from build123d import *

# Parameters (mm, degrees)
WYCI_GNI_CIE1_DEPTH        = 62
SZKIC2_R                   = 2.125
WYTNIJ_WYCI_GNI_CIE1_DEPTH = 21
SZKIC3_R                   = 2.7
WYTNIJ_WYCI_GNI_CIE2_DEPTH = 16
SZKIC4_W                   = 5
SZKIC4_H                   = 2
WYTNIJ_WYCI_GNI_CIE3_DEPTH = 21
SFAZOWANIE1_SIZE           = 0.5
SZKIC5_R                   = 2.5
WYTNIJ_WYCI_GNI_CIE4_DEPTH = 16
SZKIC6_R                   = 4
WYTNIJ_WYCI_GNI_CIE5_DEPTH = 5
SZKIC7_R                   = 2.5
WYTNIJ_WYCI_GNI_CIE6_DEPTH = 10


with BuildPart() as part:
    # Szkic1 → Wyciągnięcie1 (new body)
    with BuildSketch(Plane(origin=(0, 0, 0), x_dir=(0, 0, -1), z_dir=(1, 0, 0))):
        Polygon((0, 0), (0, -20), (13, -20), (13, -15), (15, -15), (15, -5), (13, -5), (13, 0), align=None)
    extrude(amount=WYCI_GNI_CIE1_DEPTH)

    # Szkic2 → Wytnij-wyciągnięcie1 (cut, through all)
    with BuildSketch(Plane(origin=(0, 0, 0), x_dir=(-1, 0, 0), z_dir=(0, 1, 0))):
        with Locations((-7.75, 0)):
            Circle(SZKIC2_R)
        with Locations((-23.25, 0)):
            Circle(SZKIC2_R)
        with Locations((-38.75, 0)):
            Circle(SZKIC2_R)
        with Locations((-54.25, 0)):
            Circle(SZKIC2_R)
    extrude(amount=-WYTNIJ_WYCI_GNI_CIE1_DEPTH, mode=Mode.SUBTRACT)

    # Szkic3 → Wytnij-wyciągnięcie2 (cut)
    with BuildSketch(Plane(origin=(0, -2, 0), x_dir=(-1, 0, 0), z_dir=(0, 1, 0))):
        with Locations((-7.75, 0)):
            Circle(SZKIC3_R)
        with Locations((-23.25, 0)):
            Circle(SZKIC3_R)
        with Locations((-38.75, 0)):
            Circle(SZKIC3_R)
        with Locations((-54.25, 0)):
            Circle(SZKIC3_R)
    extrude(amount=-WYTNIJ_WYCI_GNI_CIE2_DEPTH, mode=Mode.SUBTRACT)

    # Szkic4 → Wytnij-wyciągnięcie3 (cut, through all)
    with BuildSketch(Plane(origin=(0, 0, 0), x_dir=(-1, 0, 0), z_dir=(0, 1, 0))):
        with Locations((-59.5, -14)):
            Rectangle(SZKIC4_W, SZKIC4_H)
        with Locations((-2.5, -14)):
            Rectangle(SZKIC4_W, SZKIC4_H)
    extrude(amount=-WYTNIJ_WYCI_GNI_CIE3_DEPTH, mode=Mode.SUBTRACT)

    # Sfazowanie1
    sfazowanie1_edges = [part.edges().sort_by_distance(p)[0] for p in [
        (31, -5, -15),
        (31, -15, -15),
        (57, -10, -15),
        (31, 0, -13),
        (62, -10, -13),
        (31, -20, -13),
        (5, -10, -15),
        (0, -10, -13),
    ]]
    chamfer(sfazowanie1_edges, length=SFAZOWANIE1_SIZE)

    # Szkic5 → Wytnij-wyciągnięcie4 (cut, through all)
    with BuildSketch(Plane.XY):
        with Locations((31, -10)):
            Circle(SZKIC5_R)
        with Locations((46.5, -10)):
            Circle(SZKIC5_R)
        with Locations((15.5, -10)):
            Circle(SZKIC5_R)
    extrude(amount=-WYTNIJ_WYCI_GNI_CIE4_DEPTH, mode=Mode.SUBTRACT)

    # Szkic6 → Wytnij-wyciągnięcie5 (cut)
    with BuildSketch(Plane.XY):
        with Locations((46.5, -10)):
            Circle(SZKIC6_R)
        with Locations((31, -10)):
            Circle(SZKIC6_R)
        with Locations((15.5, -10)):
            Circle(SZKIC6_R)
    extrude(amount=-WYTNIJ_WYCI_GNI_CIE5_DEPTH, mode=Mode.SUBTRACT)

    # Szkic7 → Wytnij-wyciągnięcie6 (cut)
    with BuildSketch(Plane.XZ.offset(20)):
        with Locations((7.75, 0)):
            Circle(SZKIC7_R)
        with Locations((23.25, 0)):
            Circle(SZKIC7_R)
        with Locations((38.75, 0)):
            Circle(SZKIC7_R)
        with Locations((54.25, 0)):
            Circle(SZKIC7_R)
    extrude(amount=-WYTNIJ_WYCI_GNI_CIE6_DEPTH, mode=Mode.SUBTRACT)


solid = part.part
For this review, take the finished solid that the model builds, in its own axes (mm). A direction names the side the tool comes from. Give positions to 0.01 mm unless a question says otherwise; leave off trailing zeros. Order: outer loops, then holes, each group sorted by start corner. A loop starts at its lowest first (then second) coordinate and runs counter-clockwise, first axis right, second up. Notation, with made-up numbers: (85.25, 87.5) - (137.25, 87.5) arc R24 cw to (137.25, 126.5) - close; hole circle Ø7 at (40.5, -22.75). An arc over 180 degrees is marked (long way). Answer as a JSON object with one key per item and string values. Group by question number.
Item 1: Take a section at B-B on x = 15.5. Give the boundary of the cut face in (y, z), and give its area (4 significant figures).
Item 2: Take a section at A-A on z = -9.25. Give the boundary of the cut face in (x, y).
Item 3: Clearance check with flat-ended pins moving along their axes: pin 1 Ø0.8 at (y, z) = (-10, -13.5) entering from +X; pin 2 Ø1.6 at (x, z) = (35, -13.5) entering from +Y; pin 3 Ø2 at (x, z) = (23, -1) entering from -Y. State where each tip first meets the part, or that it passes through.
Item 4: Take a section at D-D on x = 54.25. Give the boundary of the cut face in (y, z) (3 decimals), and give its area (3 significant figures).
Item 5: Take a section at C-C on y = -16. Give the boundary of the cut face in (x, z), and give its area (3 significant figures).
Item 6: Wall thickness on line 1 along Y through (x, z) = (15.5, -3.6); line 2 along Y through (x, z) = (31, -8.75); line 3 along Z through (x, y) = (16, -13.5): over which ranges is each line inside the solid? List them lowest first.
Item 7: Machinability: for faces 5 (the flat face through (46, -13, -5)), 6 (the cylindrical face through (38.7, -19, -2.5)), 7 (the cylindrical face through (54.297, -0.986, -2.124)), which of the approach directions +Z, -Z, +X, -X, +Y, -Y give a long, thin tool a straight path to every point of the face, cutting with its end or side? Answer none if there is none.
Item 8: Draft analysis for pull direction X (two halves, no side actions). For faces 1 (the flat face through (19.2, -7.6, 0)), 2 (the flat face through (62, -10, -6)), 3 (the cylindrical face through (27.8, -12.4, -2.5)), 4 (the cylindrical face through (12.3, -12.4, -2.5)), state which applies: pulls with the +X half, pulls with the -X half, needs draft (parallel to the pull), parting line crosses it, or undercut.
Reported:
{
 "1": {"outline": "(-20, -12.5) - (-19.5, -13) - (-15, -13) - (-15, -14.5) - (-14.5, -15) - (-12.5, -15) - (-12.5, -5) - (-14, -5) - (-14, 0) - (-20, 0) - close; (-7.5, -15) - (-5.5, -15) - (-5, -14.5) - (-5, -13) - (-0.5, -13) - (0, -12.5) - (0, 0) - (-6, 0) - (-6, -5) - (-7.5, -5) - close", "area": "189.5 mm^2"},
 "2": {"outline": "(0, -20) - (62, -20) - (62, 0) - (0, 0) - close; hole circle Ø5 at (15.5, -10); hole circle Ø5 at (31, -10); hole circle Ø5 at (46.5, -10)"},
 "3": {"pin 1": "x = 57", "pin 2": "y = -0.2", "pin 3": "through"},
 "4": {"outline": "(-20, -12.5) - (-19.5, -13) - (-15, -13) - (-15, -14.5) - (-14.5, -15) - (-5.5, -15) - (-5, -14.5) - (-5, -13) - (-0.5, -13) - (0, -12.5) - (0, -2.125) - (-2, -2.125) - (-2, -2.7) - (-18, -2.7) - (-18, -2.5) - (-20, -2.5) - close", "area": "227 mm^2"},
 "5": {"outline": "(0, -12.5) - (0.5, -13) - (61.5, -13) - (62, -12.5) - (62, 0) - (56.95, 0) arc R2.7 cw to (51.55, 0) - (41.45, 0) arc R2.7 cw to (36.05, 0) - (25.95, 0) arc R2.7 cw to (20.55, 0) - (10.45, 0) arc R2.7 cw to (5.05, 0) - (0, 0) - close", "area": "760 mm^2"},
 "6": {"line 1": "-20 to -14, -6 to 0", "line 2": "-20 to -12.5, -7.5 to 0", "line 3": "-15 to -5"},
 "7": {"face 5": "+Z", "face 6": "+Z, -Y", "face 7": "+Z, +Y, -Y"},
 "8": {"face 1": "needs draft", "face 2": "pulls with the +X half", "face 3": "undercut", "face 4": "undercut"}
}
